Geometry check sheet. Reference: drawing and pictorial views, mm from the part's lowest x, y, z. Round coordinates to 2 decimals unless told otherwise and drop trailing zeros. Order: outer loops, then holes, each group sorted by start corner. A loop starts at its lowest first (then second) coordinate and runs counter-clockwise, first axis right, second up. Notation, with made-up numbers: M 6,8.5 L 30,8.5 A14 ccw 30,13.5 Z; hole C -9,-14 d4. An arc over 180 degrees is marked long. Answer as a JSON object with one key per item and string values. Group by question number.
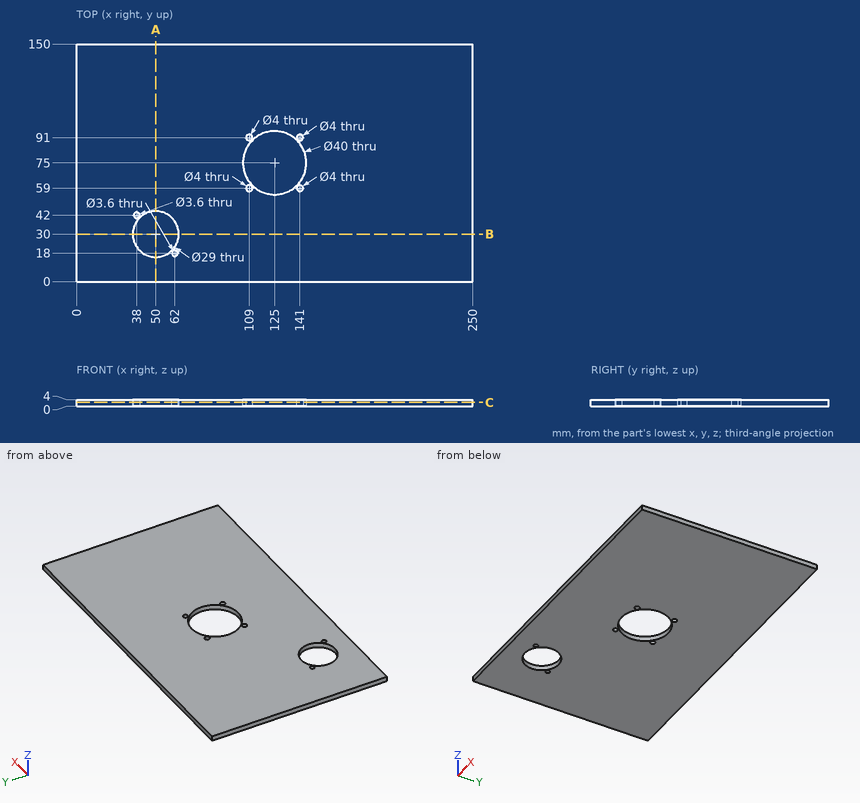
Q1. Cross-section at B-B, the plane y = 30. Record the cut outline in (x, z), then the cut area to 3 significant figures.
Q2. Gauge pin test, flat end, axial feed: pin 1 Ø12 at (x, y) = (139.5, 74) entering from -Z. Record the tip position at first contact, or that the pin passes through.
Q3. Cross-section at A-A, the plane x = 50. Record the cut outline in (y, z), then the cut area to 3 significant figures.
Q4. Cross-section at C-C, the plane z = 2.3. Give the number of separate pieces and of enclosed holes in the cut face, then the cut area to 3 significant figures.
Q5. Thickness scan on line 1 (Y direction, x = 50, z = 2.65); line 2 (Y direction, x = 109, z = 3); line 3 (Y direction, x = 38, z = 1.15). Record the ranges inside material, lowest first. Write a range as from..to.
Conclusion:
{
 "1": {"outline": "M 0,0 L 35.5,0 L 35.5,4 L 0,4 Z; M 64.5,0 L 250,0 L 250,4 L 64.5,4 Z", "area": "884 mm2"},
 "2": {"pin 1": "z = 0"},
 "3": {"outline": "M 0,0 L 15.5,0 L 15.5,4 L 0,4 Z; M 44.5,0 L 150,0 L 150,4 L 44.5,4 Z", "area": "484 mm2"},
 "4": {"separate pieces": "1", "enclosed holes": "8", "area": "35,500 mm2"},
 "5": {"line 1": "0..15.5, 44.5..150", "line 2": "0..57, 61..63, 87..89, 93..150", "line 3": "0..21.86, 38.14..40.2, 43.8..150"}
}
